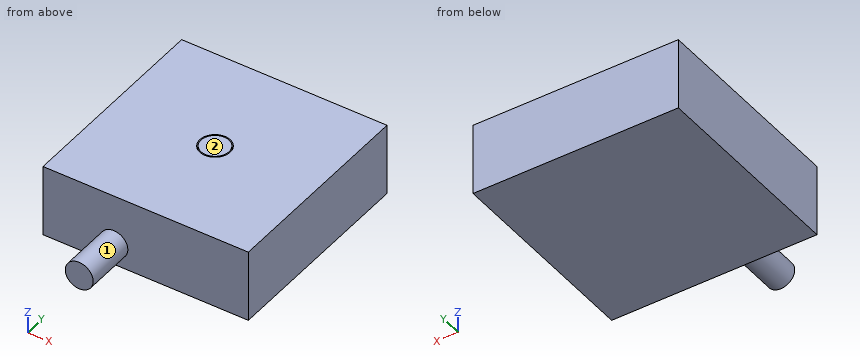
from build123d import *

# Parameters (mm, degrees)
F2_W     = 1000
F2_H     = 1000
F3_DEPTH = 350
F0_W     = 6
F0_H     = 500
F5_R     = 68
F6_DEPTH = 250


with BuildPart() as f3:
    # F2 (on offset) → F3 (new body)
    with BuildSketch(Plane.XY.offset(165.3)):
        Rectangle(F2_W, F2_H)
    extrude(amount=F3_DEPTH)

    # F0 (on Front) → F4 (revolve, cut)
    with BuildSketch(Plane.XZ):
        with Locations((-71.2, 495)):
            Rectangle(F0_W, F0_H)
    revolve(axis=Axis((0, 0, 278.492689), (0, 0, 1)), mode=Mode.SUBTRACT)

    # F5 (on face) → F6 (join)
    with BuildSketch(Plane.XZ.offset(500)):
        with Locations((-154.8, 270)):
            Circle(F5_R)
    extrude(amount=F6_DEPTH)


solid = f3.part
Source: CAD feature listing. Evaluate the final solid. Frame: model axes, mm. Face numbers are marked on the shaded views. A direction names the side the tool comes from. Give positions to 0.01 mm unless a question says otherwise; leave off trailing zeros. Loops run counter-clockwise (first coordinate to the right, second up) from the corner with the lowest first, then second, coordinate; pieces in that order, holes last. Notation, with made-up numbers: (32.25, 27) -> (89.25, 27) arc R22 cw to (89.25, 46) -> close; hole circle Ø11 at (-20, 42). An arc over 180 degrees is marked (long way). Use a Markdown table: item, result. Add a question column.
1) Line query: line 1 along Y through (x, z) = (0, 404); line 2 along X through (y, z) = (-13, 286). Output: solid intervals per line, ascending. Write a range as [from, to].
2) Reachability of the marked faces 1 and 2 from +Z, -Z, +X, -X, +Y, -Y: full face, straight path, thin tool, end or side. Return the list, or none.
3) First-contact query: pin 1 (5 mm diameter, centred on y = -536.5, z = 331.5, fed in from -X); pin 2 (4 mm diameter, centred on x = -32.5, z = 223, fed in from -Y). Flat tips, straight axial feed; report the tip coordinate or a pass-through.
4) Section query C-C, the plane z = 469.5. Return the cut outline in (x, y).
5) Section query B-B, the plane x = -154.8. Return the cut outline in (y, z), then the cut area to 3 significant figures.
6) Section query A-A, the plane z = 270. Return the cut outline in (x, y).
7) Section query D-D, the plane y = -557.5. Return the cut outline in (x, z), then the cut area to 3 significant figures.
Numbers:
| question | item | result |
|---|---|---|
| 1 | line 1 | y = [-500, -74.2], [-68.2, 68.2], [74.2, 500] |
| 1 | line 2 | x = [-500, -73.05], [-66.95, 66.95], [73.05, 500] |
| 2 | face 1 | -Y |
| 2 | face 2 | +Z, +X, -X, +Y, -Y |
| 3 | pin 1 | stops at x = -188.61 |
| 3 | pin 2 | stops at y = -500 |
| 4 | outline | (-500, -500) -> (500, -500) -> (500, 500) -> (-500, 500) -> close; circle Ø136.4 at (0, 0); hole circle Ø148.4 at (0, 0) |
| 5 | outline | (-750, 202) -> (-500, 202) -> (-500, 165.3) -> (500, 165.3) -> (500, 515.3) -> (-500, 515.3) -> (-500, 338) -> (-750, 338) -> close |
| 5 | area | 384,000 mm2 |
| 6 | outline | (-500, -500) -> (-222.8, -500) -> (-222.8, -750) -> (-86.8, -750) -> (-86.8, -500) -> (500, -500) -> (500, 500) -> (-500, 500) -> close; circle Ø136.4 at (0, 0); hole circle Ø148.4 at (0, 0) |
| 7 | outline | circle Ø136 at (-154.8, 270) |
| 7 | area | 14,500 mm2 |
